Could you check a few things on this model? Use its own coordinates, in mm. Face numbers are marked on the shaded views. Round coordinates to 2 decimals unless told otherwise and drop trailing zeros. Loops run counter-clockwise (first coordinate to the right, second up) from the corner with the lowest first, then second, coordinate; pieces in that order, holes last.
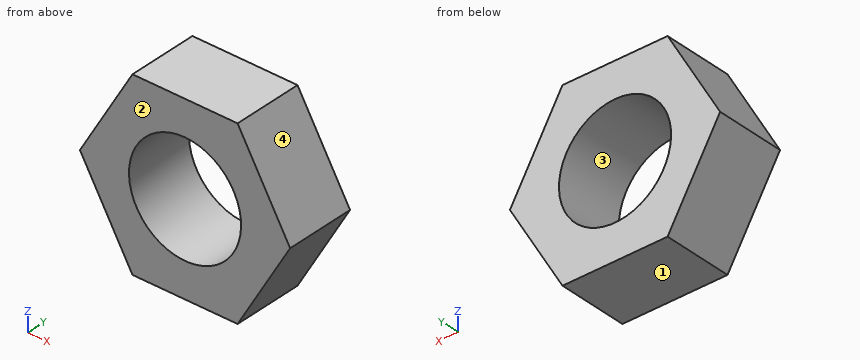
Autodesk Inventor part; units mm, degrees
ref_plane "YZ Plane" through (0, 0, 0) normal (1, 0, 0) x (0, 1, 0)
ref_plane "XZ Plane" through (0, 0, 0) normal (0, 1, 0) x (-1, 0, 0)
ref_plane "XY Plane" through (0, 0, 0) normal (0, 0, 1) x (1, 0, 0)
sketch "Sketch1" plane through (0, 0, 0) normal (0, 1, 0) x (-1, 0, 0)
  line L0 (4.7625, 0) -> (2.3813, -4.1244)
  line L1 (2.3813, -4.1244) -> (-2.3812, -4.1244)
  line L2 (-2.3812, -4.1244) -> (-4.7625, 0)
  line L3 (-4.7625, 0) -> (-2.3813, 4.1244)
  line L4 (-2.3813, 4.1244) -> (2.3812, 4.1244)
  line L5 (2.3812, 4.1244) -> (4.7625, 0)
  point P0 (0, 0)
  point P1 (0, 0)
extrude "Extrusion1" add sketch "Sketch1" along normal blind 3.175
sketch "Sketch2" plane through (0, 3.175, 0) normal (0, 1, 0) x (1, 0, 0)
  circle A0 centre (0, 0) radius 2.54
  dimension "d3" = 5.08
hole "Hole1" at (0, 3.175, 0) direction (0, -1, 0) diameter 5.08 end through all
thread "Thread1"
properties part number "Nut"
Item 1: We'd pull the mould along Z, two halves only. Please class the marked faces 1, 2, 3 and 4: released by +Z, released by -Z, zero draft, split by the parting line, or undercut.
Results list:
face 1: released by -Z
face 2: zero draft
face 3: undercut
face 4: released by +Z
Item 2: If we section it at B-B, the plane z = -1.25: Please give me the cut outline in (x, y) (3 decimals), then the cut area to 3 significant figures.
Results list:
outline: (-4.041, 0) - (-2.211, 0) - (-2.211, 3.175) - (-4.041, 3.175) - close; (2.211, 0) - (4.041, 0) - (4.041, 3.175) - (2.211, 3.175) - close
area: 11.6 mm2
Item 3: If we section it at C-C, the plane y = 2: Please give me the cut outline in (x, z), then the cut area to 3 significant figures.
Results list:
outline: (-4.76, 0) - (-2.38, -4.12) - (2.38, -4.12) - (4.76, 0) - (2.38, 4.12) - (-2.38, 4.12) - close; hole circle Ø5.08 at (0, 0)
area: 38.7 mm2
Item 4: If I drill on line 1 along Z through (x, y) = (0, 2.35); line 2 along X through (y, z) = (1.7, -2); line 3 along X through (y, z) = (2.45, -1.25), over which ranges is the centre line in solid material (lowest first)?
Results list:
line 1: z = -4.12 to -2.54, 2.54 to 4.12
line 2: x = -3.61 to -1.57, 1.57 to 3.61
line 3: x = -4.04 to -2.21, 2.21 to 4.04
Item 5: If we section it at D-D, the plane x = 4.25: Please give me the cut outline in (y, z) (3 decimals), then the cut area to 3 significant figures.
Results list:
outline: (0, -0.888) - (3.175, -0.888) - (3.175, 0.888) - (0, 0.888) - close
area: 5.64 mm2
Item 6: Will these pins go through, and if not, where does the flat tip stop? pin 1 (1.5 mm diameter, centred on y = 2, z = 3.5, fed in from +X); pin 2 (1 mm diameter, centred on x = 1, z = 3, fed in from -Y).
Results list:
pin 1: stops at x = 3.17
pin 2: stops at y = 0
Item 7: If we section it at A-A, the plane x = 0: Please give me the cut outline in (y, z) (3 decimals).
Results list:
outline: (0, -4.124) - (3.175, -4.124) - (3.175, -2.54) - (0, -2.54) - close; (0, 2.54) - (3.175, 2.54) - (3.175, 4.124) - (0, 4.124) - close
